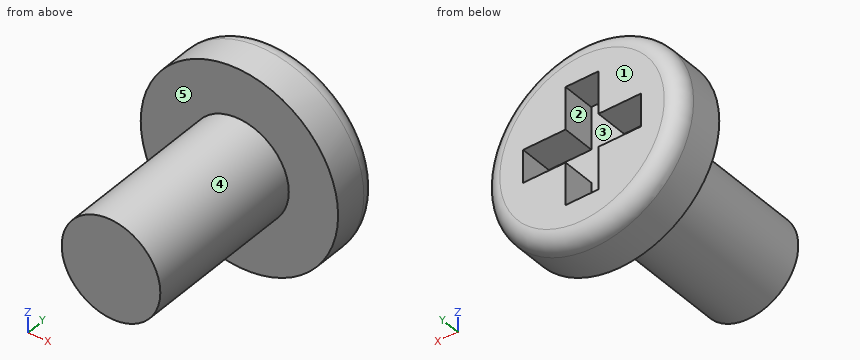
from build123d import *

# Parameters (mm, degrees)
CUT_EXTRUDE2_DEPTH = 1


with BuildPart() as part:
    # Sketch3 → Revolve1 (revolve)
    with BuildSketch(Plane.XY, mode=Mode.PRIVATE) as revolve1_sk:
        with BuildLine():
            Line((-1.5, 1.75), (-1.5, -3.25))
            Line((-1.5, -3.25), (0, -3.25))
            Line((0, -3.25), (0, 3.25))
            Line((0, 3.25), (-2.5, 3.25))
            ThreePointArc((-2.5, 3.25), (-2.853553391, 3.103553391), (-3, 2.75))
            Line((-3, 2.75), (-3, 1.75))
            Line((-3, 1.75), (-1.5, 1.75))
        make_face()
    revolve(revolve1_sk.sketch.rotate(Axis((0, -3.25, 0), (0, 1, 0)), 180), axis=Axis((0, -3.25, 0), (0, 1, 0)))

    # Sketch5 → Cut-Extrude2 (cut)
    with BuildSketch(Plane(origin=(0, 3.25, 0), x_dir=(1, 0, 0), z_dir=(0, 1, 0))):
        Polygon((-0.5, 1.790322581), (0.5, 1.790322581), (0.5, 0.5), (1.790322581, 0.5), (1.790322581, -0.5), (0.5, -0.5), (0.5, -1.790322581), (-0.5, -1.790322581), (-0.5, -0.5), (-1.790322581, -0.5), (-1.790322581, 0.5), (-0.5, 0.5), align=None)
    extrude(amount=-CUT_EXTRUDE2_DEPTH, mode=Mode.SUBTRACT)


solid = part.part
Source: CAD feature listing. Evaluate the final solid. Frame: model axes, mm. Face numbers are marked on the shaded views. A direction names the side the tool comes from. Round coordinates to 2 decimals unless told otherwise and drop trailing zeros. Write each loop counter-clockwise with the first axis right and the second up, starting at its lowest first coordinate (ties: lowest second). Pieces come first, ordered by that corner, then holes. Notation, with made-up numbers: M 26.25,27.25 L 47.25,27.25 A16 cw 47.25,42.25 Z; hole C -17,76.5 d8. An arc over 180 degrees is marked long. One line per item, written item: value. Start each with the question number.
Item 1: Section query C-C (y = -1.75). Return the cut outline in (x, z), plus the area to 3 significant figures.
Item 2: Section query A-A (x = 0). Return the cut outline in (y, z).
Item 3: Section query B-B (z = 0). Return the cut outline in (x, y), plus the area to 3 significant figures.
Item 4: Pin query (flat end, axial travel): pin 1 (1 mm diameter, centred on x = 0.5, y = 0.5, fed in from -Z); pin 2 (0.8 mm diameter, centred on x = -1, y = 2.5, fed in from +Z); pin 3 (0.5 mm diameter, centred on x = 1, y = 3, fed in from -Z); pin 4 (0.5 mm diameter, centred on y = 3, z = 0, fed in from +X). Return the tip coordinate at first contact, or that it passes through.
Item 5: Ray query, L1, parallel to Y at x = -1, z = 0; L2, parallel to X at y = 2.75, z = -1; L3, parallel to X at y = 3, z = 0.25. Return the intervals inside material, ascending. Write a range as from..to.
Item 6: Set-up query: the marked faces 1 and 2. Return all of +Z, -Z, +X, -X, +Y, -Y with unobstructed straight access to the full face (end or side cutting, diameter ignored); none if empty.
Item 7: Mould query, pull axis X, two halves, no side actions, for the marked faces 3, 4 and 5. Classes: pulls with the +X half, pulls with the -X half, needs draft (parallel to the pull), parting line crosses it, or undercut.
Result set:
1. outline: C 0,0 d3
1. area: 7.07 mm²
2. outline: M -3.25,-1.5 L 1.75,-1.5 L 1.75,-3 L 2.75,-3 A0.5 ccw 3.25,-2.5 L 3.25,-1.79 L 2.25,-1.79 L 2.25,1.79 L 3.25,1.79 L 3.25,2.5 A0.5 ccw 2.75,3 L 1.75,3 L 1.75,1.5 L -3.25,1.5 Z
3. outline: M -3,1.75 L -1.5,1.75 L -1.5,-3.25 L 1.5,-3.25 L 1.5,1.75 L 3,1.75 L 3,2.75 A0.5 ccw 2.5,3.25 L 1.79,3.25 L 1.79,2.25 L -1.79,2.25 L -1.79,3.25 L -2.5,3.25 A0.5 ccw -3,2.75 Z
3. area: 20.3 mm²
4. pin 1: stops at z = -1.5
4. pin 2: stops at z = 2.94
4. pin 3: stops at z = -2.88
4. pin 4: stops at x = 3
5. L1: y = -3.25..2.25
5. L2: x = -2.83..-0.5, 0.5..2.83
5. L3: x = -2.92..-1.79, 1.79..2.92
6. face 1: +Z, -Z, +X, -X, +Y
6. face 2: +Y
7. face 3: undercut
7. face 4: parting line crosses it
7. face 5: needs draft
